Build history of the part. All positions in model axes, mm. Face numbers are marked on the shaded views. A direction names the side the tool comes from. Round coordinates to 2 decimals unless told otherwise and drop trailing zeros. Loops run counter-clockwise (first coordinate to the right, second up) from the corner with the lowest first, then second, coordinate; pieces in that order, holes last. Notation, with made-up numbers: (79.5, 46.5) -> (97.5, 46.5) arc R16 ccw to (97.5, 71.5) -> close; hole circle Ø9 at (78, 55). An arc over 180 degrees is marked (long way). Put each result on its own line as item: value. Start each with the question number.
Item 1: Cut at B-B, the plane x = 0. List the corners of the cut face in (y, z).
Item 2: Flat gauge pins, fed straight in: pin 1 Ø12 at (x, y) = (2.5, 5) entering from +Z; pin 2 Ø0.6 at (x, y) = (-11, 6) entering from -Z; pin 3 Ø1.5 at (y, z) = (-2.5, 6.5) entering from -X. Where does each tip first touch, or does it go through?
Item 3: Tool access for the marked faces 1 and 2: list every direction of +Z, -Z, +X, -X, +Y, -Y with a clear straight run to the whole face (end or side of a thin tool).
Item 4: Drill centre lines: probe 1 along Y at (x, z) = (0, -1.25); probe 2 along X at (y, z) = (4, 6.25); probe 3 along Y at (x, z) = (0, 3). Where is each one in solid material? Low to high. Write a range as [from, to].
Item 5: Cut at A-A, the plane y = 4. List the corners of the cut face in (x, z), plus the area to 3 significant figures.
Item 6: Pull direction X, two halves, no side cores. Call the marked faces 3, 4, 5 and 6: +X half, -X half, draft (parallel to the pull), parting line (faces both ways), or undercut.
Item 7: Cut at C-C, the plane z = 19.5. List the corners of the cut face in (x, y), plus the area to 3 significant figures.
Item 8: Cut at D-D, the plane x = 6.5. List the corners of the cut face in (y, z), plus the area to 3 significant figures.
Autodesk Inventor part; units mm, degrees
ref_plane "YZ Plane" through (0, 0, 0) normal (1, 0, 0) x (0, 1, 0)
ref_plane "XZ Plane" through (0, 0, 0) normal (0, 1, 0) x (-1, 0, 0)
ref_plane "XY Plane" through (0, 0, 0) normal (0, 0, 1) x (1, 0, 0)
sketch "Sketch1" plane through (0, 0, 0) normal (0, 0, 1) x (1, 0, 0)
  line L0 (-10, -17.5) -> (10, -17.5)
  line L1 (10, -17.5) -> (10, 17.5)
  line L2 (10, 17.5) -> (-10, 17.5)
  line L3 (-10, 17.5) -> (-10, -17.5)
  line L4 (-10, -17.5) -> (10, 17.5) construction
  line L5 (10, -17.5) -> (-10, 17.5) construction
  point P0 (0, 0)
  dimension "d0" = 20
  dimension "d1" = 35
extrude "Extrusion1" add sketch "Sketch1" along normal blind 40
sketch "Sketch2" plane through (0, 0, 40) normal (0, 0, 1) x (1, 0, 0)
  line L0 (-8, -16) -> (8, -16)
  line L1 (8, -16) -> (8, 16)
  line L2 (8, 16) -> (-8, 16)
  line L3 (-8, 16) -> (-8, -16)
  point P0 (0, 0)
  dimension "d4" = 16
  dimension "d5" = 32
extrude "Extrusion2" cut sketch "Sketch2" against normal blind 30
sketch "Sketch3" plane through (0, 0, 10) normal (0, 0, 1) x (1, 0, 0)
  line L0 (8, -16) -> (-8, -16)
  line L1 (8, 16) -> (8, -16)
  line L2 (-8, 16) -> (8, 16)
  line L3 (-8, -16) -> (-8, 16)
  point P0 (0, 0)
sketch "Sketch5" plane through (-10, -17.5, 0) normal (-1, 0, 0) x (0, 0, 1)
  line L0 (0, 35) -> (0, 0)
  line L1 (0, 0) -> (40, 0)
  line L2 (40, 35) -> (40, 0)
  line L3 (0, 35) -> (40, 35)
  point P0 (0, 17.5)
sketch "Sketch6" plane through (-10, -17.5, 0) normal (-1, 0, 0) x (0, 0, 1)
  line L0 (0, 35) -> (0, 0)
  line L1 (0, 0) -> (40, 0)
  line L2 (0, 35) -> (40, 35)
  line L3 (0, 35) -> (5, 35)
  line L4 (5, 35) -> (5, 0)
  line L5 (5, 0) -> (0, 0)
  line L6 (0, 0) -> (0, 35)
  line L7 (40, 35) -> (35, 35)
  line L8 (35, 35) -> (35, 0)
  line L9 (35, 0) -> (40, 0)
  line L10 (40, 0) -> (40, 35)
  line L11 (10, 0) -> (30, 0)
  line L12 (30, 0) -> (30, 35)
  line L13 (30, 35) -> (10, 35)
  line L14 (10, 35) -> (10, 0)
  point P0 (0, 17.5)
  dimension "d16" = 5
  dimension "d17" = 5
  dimension "d18" = 20
extrude "Extrusion3" add sketch "Sketch6" along normal blind 2 contours L2 L4 L1 L0 | L2 L12 L1 L14 | L2 L10 L1 L8
sketch "Sketch7" plane through (0, 0, 10) normal (0, 0, 1) x (1, 0, 0)
  circle A0 centre (0, 4) radius 2.25
  point P0 (0, 0)
  dimension "d21" = 4.5
extrude "Extrusion4" cut sketch "Sketch7" against normal through all
sketch "Sketch8" plane through (0, 0, 0) normal (0, 0, -1) x (-1, 0, 0)
  circle A0 centre (0, 4) radius 2.25
  circle A1 centre (0, 4) radius 3.5
  point P0 (0, 0)
  dimension "d24" = 7
extrude "Extrusion5" add sketch "Sketch8" along normal blind 8
properties part number "atmos-pressure-end"
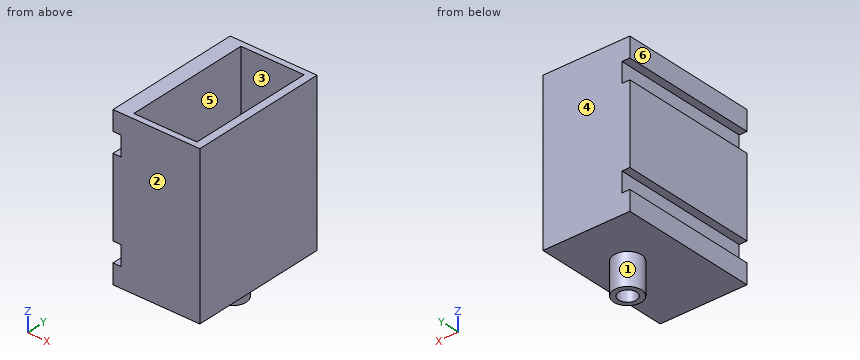
Reply:
1. outline: (-17.5, 0) -> (0.5, 0) -> (0.5, -8) -> (1.75, -8) -> (1.75, 10) -> (-16, 10) -> (-16, 40) -> (-17.5, 40) -> close; (6.25, -8) -> (7.5, -8) -> (7.5, 0) -> (17.5, 0) -> (17.5, 40) -> (16, 40) -> (16, 10) -> (6.25, 10) -> close
2. pin 1: stops at z = 40
2. pin 2: stops at z = 0
2. pin 3: stops at x = -10
3. face 1: -Z
3. face 2: +Z, -Z, +X, -X, -Y
4. probe 1: y = [0.5, 1.75], [6.25, 7.5]
4. probe 2: x = [-10, -2.25], [2.25, 10]
4. probe 3: y = [-17.5, 1.75], [6.25, 17.5]
5. outline: (-12, 0) -> (-3.5, 0) -> (-3.5, -8) -> (-2.25, -8) -> (-2.25, 10) -> (-8, 10) -> (-8, 40) -> (-12, 40) -> (-12, 35) -> (-10, 35) -> (-10, 30) -> (-12, 30) -> (-12, 10) -> (-10, 10) -> (-10, 5) -> (-12, 5) -> close; (2.25, -8) -> (3.5, -8) -> (3.5, 0) -> (10, 0) -> (10, 40) -> (8, 40) -> (8, 10) -> (2.25, 10) -> close
5. area: 355 mm^2
6. face 3: undercut
6. face 4: draft
6. face 5: undercut
6. face 6: -X half
7. outline: (-12, -17.5) -> (10, -17.5) -> (10, 17.5) -> (-12, 17.5) -> close; hole (-8, -16) -> (8, -16) -> (8, 16) -> (-8, 16) -> close
7. area: 258 mm^2
8. outline: (-17.5, 0) -> (17.5, 0) -> (17.5, 40) -> (16, 40) -> (16, 10) -> (-16, 10) -> (-16, 40) -> (-17.5, 40) -> close
8. area: 440 mm^2
